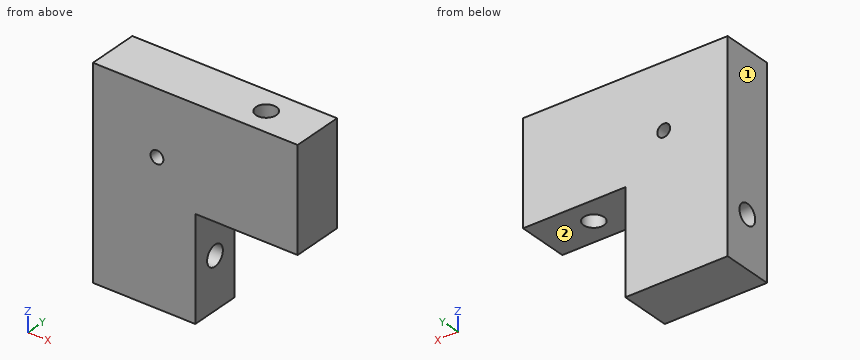
from build123d import *

# Parameters (mm, degrees)
RESSALTO_EXTRUS_O1_DEPTH = 20
ESBO_O3_R                = 4
CORTE_EXTRUS_O1_DEPTH    = 63.524475359
ESBO_O4_R                = 4
CORTE_EXTRUS_O2_DEPTH    = 84.066238629
ESBO_O5_R                = 2.5
CORTE_EXTRUS_O3_DEPTH    = 85.907655832


with BuildPart() as part:
    # Esboço1 → Ressalto-extrusão1 (new body)
    with BuildSketch(Plane(origin=(0, 0, 0), x_dir=(1, 0, 0), z_dir=(0, 1, 0))):
        Polygon((-70, 36.304347826), (-70, -43.695652174), (10, -43.695652174), (10, -3.695652174), (-30, -3.695652174), (-30, 36.304347826), align=None)
    extrude(amount=RESSALTO_EXTRUS_O1_DEPTH)

    # Esboço3 → Corte-extrusão1 (cut, through all)
    with BuildSketch(Plane(origin=(-30, 0, 0), x_dir=(0, 0, -1), z_dir=(1, 0, 0))):
        with Locations((16.304347826, 10)):
            Circle(ESBO_O3_R)
    extrude(amount=-CORTE_EXTRUS_O1_DEPTH, mode=Mode.SUBTRACT)

    # Esboço4 → Corte-extrusão2 (cut, through all)
    with BuildSketch(Plane(origin=(0, 0, 3.695652174), x_dir=(-1, 0, 0), z_dir=(0, 0, -1))):
        with Locations((10, 10)):
            Circle(ESBO_O4_R)
    extrude(amount=-CORTE_EXTRUS_O2_DEPTH, mode=Mode.SUBTRACT)

    # Esboço5 → Corte-extrusão3 (cut, through all)
    with BuildSketch(Plane.XZ):
        with Locations(Location((-45, 18.695652174, 0), (0, 0, 270))):
            Circle(ESBO_O5_R)
    extrude(amount=-CORTE_EXTRUS_O3_DEPTH, mode=Mode.SUBTRACT)


solid = part.part
Design review of the part built by this model. Coordinates are the model's own, in mm. Face numbers are marked on the shaded views. A direction names the side the tool comes from. Coordinates: 2 decimals unless noted, no trailing zeros. Loops run counter-clockwise (first coordinate to the right, second up) from the corner with the lowest first, then second, coordinate; pieces in that order, holes last. Notation, with made-up numbers: (71, 28) -> (102, 28) arc R24 ccw to (102, 53) -> close; hole circle Ø10 at (64, -34.5). An arc over 180 degrees is marked (long way). Use a Markdown table: item, result. Add a question column.
Item 1: Wall thickness on L1, parallel to Z at x = -12.5, y = 2; L2, parallel to Y at x = -63.5, z = -16; L3, parallel to Y at x = -32.5, z = -18: over which ranges is each line inside the solid? List them lowest first. Write a range as from..to.
Item 2: Clearance check with flat-ended pins moving along their axes: P1, Ø6, axis at y = 5, z = -13.5, coming from the +X side; P2, Ø4, axis at x = -45, z = 18.7, coming from the -Y side. State where each tip first meets the part, or that it passes through.
Item 3: We need section D-D, the plane y = 3.25. Write out the cut boundary in (x, z), and give its area (3 significant figures).
Item 4: We need section B-B, the plane x = -45. Write out the cut boundary in (y, z), and give its area (3 significant figures).
Item 5: Machinability: for the marked faces 1 and 2, which of the approach directions +Z, -Z, +X, -X, +Y, -Y give a long, thin tool a straight path to every point of the face, cutting with its end or side? Answer none if there is none.
Item 6: We need section A-A, the plane y = 10. Write out the cut boundary in (x, z).
Item 7: We need section C-C, the plane z = 19. Write out the cut boundary in (x, y), and give its area (3 significant figures).
Numbers:
| question | item | result |
|---|---|---|
| 1 | L1 | z = 3.7..43.7 |
| 1 | L2 | y = 0..6.01, 13.99..20 |
| 1 | L3 | y = 0..6.38, 13.62..20 |
| 2 | P1 | stops at x = -30 |
| 2 | P2 | passes through |
| 3 | outline | (-70, -36.3) -> (-30, -36.3) -> (-30, 3.7) -> (10, 3.7) -> (10, 43.7) -> (-70, 43.7) -> close; hole circle Ø5 at (-45, 18.7) |
| 3 | area | 4,780 mm^2 |
| 4 | outline | (0, -36.3) -> (20, -36.3) -> (20, 16.2) -> (0, 16.2) -> close; (0, 21.2) -> (20, 21.2) -> (20, 43.7) -> (0, 43.7) -> close; hole circle Ø8 at (10, -16.3) |
| 4 | area | 1,450 mm^2 |
| 5 | face 1 | +Z, -Z, -X, +Y, -Y |
| 5 | face 2 | -Z, +X, +Y, -Y |
| 6 | outline | (-70, -36.3) -> (-30, -36.3) -> (-30, -20.3) -> (-70, -20.3) -> close; (-70, -12.3) -> (-30, -12.3) -> (-30, 3.7) -> (-14, 3.7) -> (-14, 43.7) -> (-70, 43.7) -> close; (-6, 3.7) -> (10, 3.7) -> (10, 43.7) -> (-6, 43.7) -> close; hole circle Ø5 at (-45, 18.7) |
| 7 | outline | (-70, 0) -> (-47.48, 0) -> (-47.48, 20) -> (-70, 20) -> close; (-42.52, 0) -> (10, 0) -> (10, 20) -> (-42.52, 20) -> close; hole circle Ø8 at (-10, 10) |
| 7 | area | 1,450 mm^2 |
